Answer from the drawing. Dimensions are ordinates in mm from the lowest x, y and z of the part. A direction names the side the tool comes from. Coordinates: 2 decimals unless noted, no trailing zeros. Write each loop counter-clockwise with the first axis right and the second up, starting at its lowest first coordinate (ties: lowest second). Pieces come first, ordered by that corner, then holes. Notation, with made-up numbers: (8, 43) -> (13, 43) arc R28 cw to (13, 78) -> close; hole circle Ø1 at (1, 88). An arc over 180 degrees is marked (long way). One line per item, written item: value. Start each with the question number.
1. Find section A-A, the plane z = 5. Write down the section's boundary in (x, y).
2. Find section B-B, the plane x = 5. Write down the section's boundary in (y, z).
3. Given P1, Ø5, axis at x = 2, y = 5, coming from the -Z side; P2, Ø3, axis at y = 5.5, z = 3.5, coming from the +X side; P3, Ø3, axis at y = 8, z = 2.5, coming from the -X side, each flat-ended and moving along its own axis, determine where each tip first touches the part or whether it passes through.
4. Find section D-D, the plane z = 1. Write down the section's boundary in (x, y).
5. Find section C-C, the plane x = 1. Write down the section's boundary in (y, z), and give its area (3 significant figures).
6. For the marked faces 1 and 2, determine the directions among +Z, -Z, +X, -X, +Y, -Y from which every point of the face is accessible in a straight line to the end or side of a thin tool.
7. Consider line 1 along X through (y, z) = (7.5, 5); line 2 along Y through (x, z) = (1.5, 8). Determine where each line is inside the solid, lowest interval first.
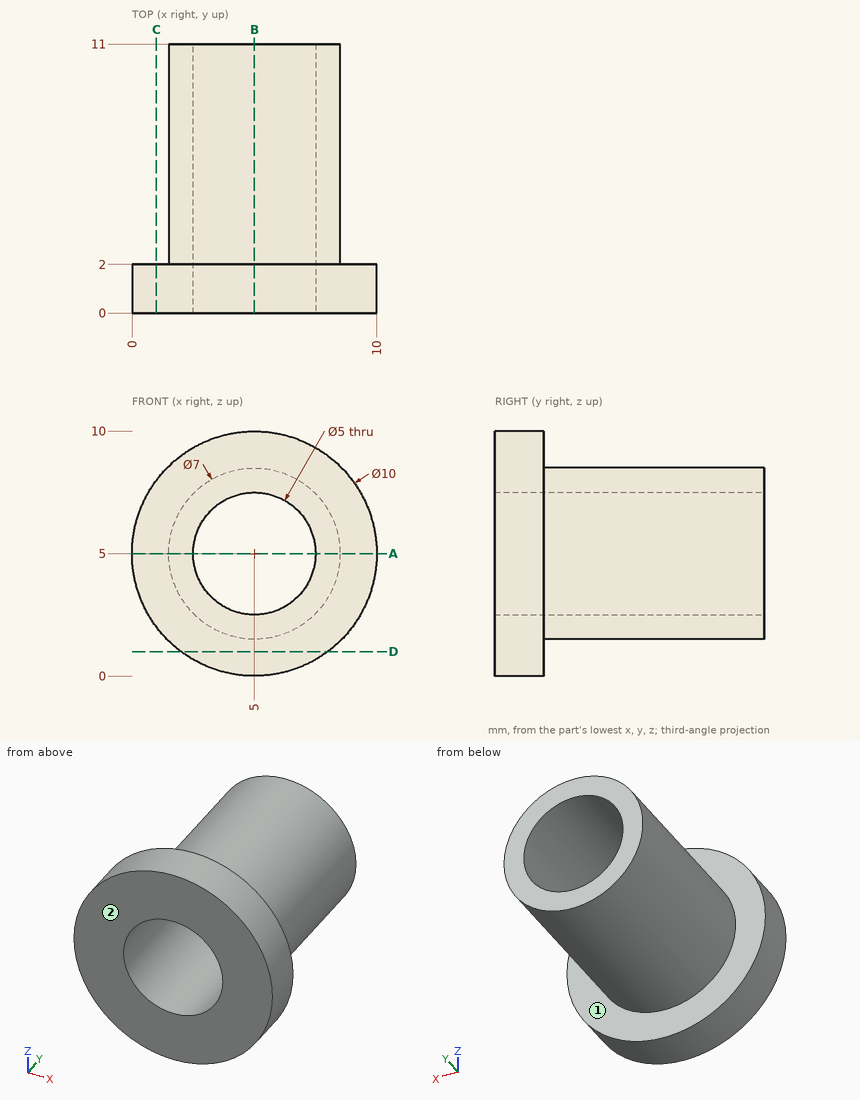
Answer block:
1. outline: (0, 0) -> (2.5, 0) -> (2.5, 11) -> (1.5, 11) -> (1.5, 2) -> (0, 2) -> close; (7.5, 0) -> (10, 0) -> (10, 2) -> (8.5, 2) -> (8.5, 11) -> (7.5, 11) -> close
2. outline: (0, 0) -> (2, 0) -> (2, 1.5) -> (11, 1.5) -> (11, 2.5) -> (0, 2.5) -> close; (0, 7.5) -> (11, 7.5) -> (11, 8.5) -> (2, 8.5) -> (2, 10) -> (0, 10) -> close
3. P1: stops at z = 1.54
3. P2: stops at x = 8.5
3. P3: stops at x = 1.65
4. outline: (2, 0) -> (8, 0) -> (8, 2) -> (2, 2) -> close
5. outline: (0, 2) -> (2, 2) -> (2, 8) -> (0, 8) -> close
5. area: 12.0 mm2
6. face 1: +Y
6. face 2: +Z, -Z, +X, -X, -Y
7. line 1: x = 1.5 to 2.5, 7.5 to 8.5
7. line 2: y = 0 to 2
